```python
from build123d import *

# Parameters (mm, degrees)
SKETCH1_W           = 5.8
SKETCH1_H           = 4.2
BOSS_EXTRUDE1_DEPTH = 7.8
CUT_EXTRUDE1_DEPTH  = 7


with BuildPart() as part:
    # Sketch1 → Boss-Extrude1 (new body)
    with BuildSketch(Plane(origin=(0, 0, 0), x_dir=(1, 0, 0), z_dir=(0, 1, 0))):
        with Locations((2.9, 2.1)):
            Rectangle(SKETCH1_W, SKETCH1_H)
    extrude(amount=BOSS_EXTRUDE1_DEPTH)

    # Sketch2 → Cut-Extrude1 (cut)
    with BuildSketch(Plane(origin=(0, 7.8, 0), x_dir=(1, 0, 0), z_dir=(0, 1, 0))):
        with BuildLine():
            Line((2.225, 0.5), (5.3, 0.5))
            Line((5.3, 0.5), (5.3, 3.7))
            Line((5.3, 3.7), (3.15, 3.7))
            Line((3.15, 3.7), (3.15, 3.4))
            Line((3.15, 3.4), (2.65, 3.4))
            Line((2.65, 3.4), (2.65, 3.7))
            Line((2.65, 3.7), (2.225, 3.7))
            ThreePointArc((2.225, 3.7), (0.625, 2.1), (2.225, 0.5))
        make_face()
    extrude(amount=-CUT_EXTRUDE1_DEPTH, mode=Mode.SUBTRACT)


solid = part.part
```
Check sheet for the modelled part. Datum: model origin and axes. Units: mm. A direction names the side the tool comes from. Round coordinates to 2 decimals unless told otherwise and drop trailing zeros. Order: outer loops, then holes, each group sorted by start corner. A loop starts at its lowest first (then second) coordinate and runs counter-clockwise, first axis right, second up. Notation, with made-up numbers: (3, 46) - (17, 46) arc R35 cw to (17, 81) - close; hole circle Ø9 at (52.5, 6.25). An arc over 180 degrees is marked (long way). Answer as CSV lines item,"result". Start each with the question number.
1) Section check B-B (z = -2.1). Record the cut outline in (x, y) (3 decimals), then the cut area to 3 significant figures.
2) Scan lines: probe 1 along Z at (x, y) = (4.2, 3.25); probe 2 along Z at (x, y) = (3, 5.25); probe 3 along Y at (x, z) = (2.45, -3.65). Record each from-to range of solid material in increasing order.
3) Tool access check on faces 4 (the face through (3, 0, -2)), 5 (the face through (4, 4, -0.5)). Record the directions out of +Z, -Z, +X, -X, +Y, -Y that give a thin tool (end or side, any length) a straight path to the whole face; none if there is none.
4) Section check C-C (x = 1.65). Record the cut outline in (y, z).
5) Depth check by flat-ended pin: pin 1 (1.6 mm diameter, centred on x = 3.5, z = -2.5, fed in from +Y). Enter the tip coordinate at first touch or a pass-through.
6) Draft check along Z on faces 1 (the face through (3, 4, 0)), 2 (the face through (5.3, 4, -2)), 3 (the face through (3, 7.8, -4)). Enter one of: +Z half, -Z half, draft (parallel to the pull), parting line (faces both ways), or undercut.
7) Section check A-A (y = 2.5). Record the cut outline in (x, z) (3 decimals).
Determined:
1,outline,"(0, 0) - (5.8, 0) - (5.8, 7.8) - (5.3, 7.8) - (5.3, 0.8) - (0.625, 0.8) - (0.625, 7.8) - (0, 7.8) - close"
1,area,"12.5 mm^2"
2,probe 1,"-4.2 to -3.7, -0.5 to 0"
2,probe 2,"-4.2 to -3.4, -0.5 to 0"
2,probe 3,"0 to 0.8"
3,face 4,"+Z, -Z, +X, -X, -Y"
3,face 5,"+Y"
4,outline,"(0, -4.2) - (7.8, -4.2) - (7.8, -3.59) - (0.8, -3.59) - (0.8, -0.61) - (7.8, -0.61) - (7.8, 0) - (0, 0) - close"
5,pin 1,"y = 0.8"
6,face 1,"+Z half"
6,face 2,"undercut"
6,face 3,"draft"
7,outline,"(0, -4.2) - (5.8, -4.2) - (5.8, 0) - (0, 0) - close; hole (2.225, -3.7) - (2.65, -3.7) - (2.65, -3.4) - (3.15, -3.4) - (3.15, -3.7) - (5.3, -3.7) - (5.3, -0.5) - (2.225, -0.5) arc R1.6 ccw to start"
